For this review, take the finished solid that the model builds, in its own axes (mm). A direction names the side the tool comes from. Give positions to 0.01 mm unless a question says otherwise; leave off trailing zeros. Write each loop counter-clockwise with the first axis right and the second up, starting at its lowest first coordinate (ties: lowest second). Pieces come first, ordered by that corner, then holes. Notation, with made-up numbers: M 89,-30.5 L 97,-30.5 A11 ccw 97,-17.5 Z; hole C 57,36 d10. An arc over 180 degrees is marked long. Use one line per item in the form item = value. Start each with the question number.
Q1. Consider section A-A on z = 0. Give the number of separate pieces and of enclosed holes in the cut face, and give its area (3 significant figures).
Q2. Mouldability with a two-part tool opening along Z and no side actions: class faces 5 (the flat face through (-10.905, 13, 13)), 6 (the cylindrical face through (-1.17, -16.855, -2.213)), 7 (the cylindrical face through (-0.209, -3.604, 11.446)) as released by +Z, released by -Z, zero draft, split by the parting line, or undercut.
Q3. Clearance check with flat-ended pins moving along their axes: pin 1 Ø6 at (x, z) = (-11.5, -20) entering from +Y; pin 2 Ø1 at (x, z) = (-3.5, -15.5) entering from -Y; pin 3 Ø2 at (x, y) = (7.5, -10) entering from -Z. State where each tip first meets the part, or that it passes through.
Q4. Consider section D-D on z = -26. Write out the cut boundary in (x, y), and give its area (3 significant figures).
Q5. For probe 1 along Y at (x, z) = (-13.05, 0); probe 2 along X at (y, z) = (-25, -15.5); probe 3 along Z at (x, y) = (-13, -2.5), list the stretches that pass through material, from the lowest coordinate up. Write a range as [from, to].
Q6. Consider section C-C on x = -12.25. Write out the cut boundary in (y, z).
Q7. Tool access review of faces 1 (the flat face through (13.33, -13, 17)), 2 (the flat face through (14.905, 9, 9)), 3 (the cylindrical face through (-12.933, 28.727, 0.358)), 4 (the conical face through (9.54, 16.17, 8.41)): name each direction out of +Z, -Z, +X, -X, +Y, -Y from which nothing blocks a thin tool from reaching the whole face with its end or side.
```python
from build123d import *

# Parameters (mm, degrees)
M5_START                     = -14.904727216
M5_CLEARANCE_HOLE1_OUTLINE_R = 2.75
M5_CLEARANCE_HOLE1_DEPTH     = 4
CIRPATTERN1_COUNT            = 4


# Read off the part's stored shape, not the designer's step: M5 Clearance Hole1
with BuildPart() as part:
    # Sketch1 → Revolve1 (revolve)
    with BuildSketch(Plane.XY, mode=Mode.PRIVATE) as revolve1_sk:
        with BuildLine():
            Line((-14.904727216, 12), (-14.904727216, 31))
            Line((-14.904727216, 31), (-10.904727216, 31))
            Line((-10.904727216, 31), (-10.904727216, 17))
            Line((-10.904727216, 17), (8.294935567, 17))
            ThreePointArc((8.294935567, 17), (8.950533434, 17.206709213), (9.369004233, 17.752070976))
            Line((9.369004233, 17.752070976), (12.098027216, 25.25))
            Line((12.098027216, 25.25), (14.904727216, 25.25))
            Line((14.904727216, 25.25), (14.904727216, 23.1186))
            Line((14.904727216, 23.1186), (13.329927216, 22.450137059))
            Line((13.329927216, 22.450137059), (13.329927216, 21.187062941))
            Line((13.329927216, 21.187062941), (14.904727216, 20.5186))
            Line((14.904727216, 20.5186), (14.904727216, 12))
            Line((14.904727216, 12), (-14.904727216, 12))
        make_face()
    revolve(revolve1_sk.sketch.rotate(Axis((0, 0, 0), (1, 0, 0)), 90), axis=Axis((0, 0, 0), (1, 0, 0)))

    # M5 Clearance Hole1 outline → M5 Clearance Hole1 (cut)
    with BuildSketch(Plane.YZ.offset(M5_START)):
        with Locations((0, 26)):
            Circle(M5_CLEARANCE_HOLE1_OUTLINE_R)
    m5_clearance_hole1 = extrude(amount=M5_CLEARANCE_HOLE1_DEPTH, mode=Mode.SUBTRACT)

    # CirPattern1: M5 Clearance Hole1 ×4 about axis
    cirpattern1_axis = Axis((0, 0, 0), (1, 0, 0))
    for i in range(1, CIRPATTERN1_COUNT):
        add(m5_clearance_hole1.rotate(cirpattern1_axis, i * 360 / CIRPATTERN1_COUNT), mode=Mode.SUBTRACT)


solid = part.part
```
Working result:
q1.separate_pieces = 4
q1.enclosed_holes = 0
q1.area = 431 mm²
q2.face_5 = zero draft
q2.face_6 = split by the parting line
q2.face_7 = undercut
q3.pin_1 = 25.92
q3.pin_2 = -8
q3.pin_3 = -14.42
q4.outline = M -14.9,-16.88 L -10.9,-16.88 L -10.9,-2.75 L -14.9,-2.75 Z; M -14.9,2.75 L -10.9,2.75 L -10.9,16.88 L -14.9,16.88 Z
q4.area = 113 mm²
q5.probe_1 = [-31, -28.75], [-23.25, -12], [12, 23.25], [28.75, 31]
q5.probe_2 = [-14.9, -10.9]
q5.probe_3 = [-30.9, -27.15], [-24.85, -11.74], [11.74, 24.85], [27.15, 30.9]
q6.outline = C 0,0 d62; hole C -26,0 d5.5; hole C 0,0 d24; hole C 0,-26 d5.5; hole C 0,26 d5.5; hole C 26,0 d5.5
q7.face_1 = +X
q7.face_2 = +Z, -Z, +X, +Y, -Y
q7.face_3 = -X
q7.face_4 = none
